from build123d import *

# Parameters (mm, degrees)
BOSS_EXTRUDE1_DEPTH = 4.7625
CUT_EXTRUDE1_DEPTH  = 3.175
FILLET1_R           = 3.302
SKETCH3_R           = 31.75
CUT_EXTRUDE2_DEPTH  = 12.7
CHAMFER1_SIZE       = 2.23064129
CHAMFER1_SIZE_2     = 2.54
SKETCH4_R           = 1.55
CUT_EXTRUDE3_DEPTH  = 50.289254661


with BuildPart() as part:
    # Sketch1 → Boss-Extrude1 (new, symmetric)
    with BuildSketch(Plane.XY):
        Polygon((-44.45, 19.05), (-44.45, -6.35), (-25.4, -6.35), (-25.4, 6.35), (-28.575, 6.35), (-28.575, 19.05), align=None)
    extrude(amount=BOSS_EXTRUDE1_DEPTH, both=True)

    # Sketch2 → Cut-Extrude1 (cut, symmetric)
    with BuildSketch(Plane.XY):
        Polygon((-44.45, 19.05), (-38.1, 19.05), (-38.1, 0), (-25.4, 0), (-25.4, -6.35), (-44.45, -6.35), align=None)
    extrude(amount=CUT_EXTRUDE1_DEPTH, both=True, mode=Mode.SUBTRACT)

    # Fillet1
    fillet1_edges = [part.edges().sort_by_distance(p)[0] for p in [
        (-38.1, 0, 0),
    ]]
    fillet(fillet1_edges, radius=FILLET1_R)

    # Sketch3 → Cut-Extrude2 (cut)
    with BuildSketch(Plane(origin=(0, 19.05, 0), x_dir=(1, 0, 0), z_dir=(0, 1, 0))):
        Circle(SKETCH3_R)
    extrude(amount=-CUT_EXTRUDE2_DEPTH, mode=Mode.SUBTRACT)

    # Chamfer1
    # the kernel refuses this chamfer: 2.54, 2.23064129 mm, written as the material it takes off along each edge
    with BuildSketch(Plane(origin=(-31.390780394, 6.35, -4.7625), x_dir=(-1, 0, 0), z_dir=(0, 1, 0))) as chamfer1_piece_1:
        with BuildLine():
            Line((CHAMFER1_SIZE, 0), (0.288027051, 2.637492029))
            ThreePointArc((0.288027051, 2.637492029), (0.17562072, 1.352980867), (0, 0))
            Line((0, 0), (CHAMFER1_SIZE, 0))
        make_face()
    extrude(amount=19.52205078, mode=Mode.SUBTRACT)
    with BuildSketch(Plane(origin=(-31.390780394, 6.35, 4.7625), x_dir=(-0.11419845391674416, 0, -0.993457957400828), z_dir=(0, 1, 0))) as chamfer1_piece_2:
        with BuildLine():
            Line((2.293129868, 0), (CHAMFER1_SIZE_2 * 0.114198453917, CHAMFER1_SIZE_2 * 0.993457957401))
            Line((CHAMFER1_SIZE_2 * 0.114198453917, CHAMFER1_SIZE_2 * 0.993457957401), (0, 0))
            ThreePointArc((0, 0), (1.178209116, 0.020693522), (2.293129868, 0))
        make_face()
    extrude(amount=19.232074789, mode=Mode.SUBTRACT)
    with BuildSketch(Plane(origin=(0, 19.05, 0), x_dir=(-0.9371917542835735, 0, -0.34881458642504903), z_dir=(0.34881458642504903, 0, -0.9371917542835735))) as chamfer1_piece_3:
        Polygon((31.75, -CHAMFER1_SIZE_2), (31.75 + CHAMFER1_SIZE_2, 0), (31.75, 0), align=None)
    revolve(axis=Axis((0, 19.05, 0), (0, 1, 0)), revolution_arc=40.829654119, mode=Mode.SUBTRACT)

    # Sketch4 → Cut-Extrude3 (cut, through all)
    with BuildSketch(Plane.XY.offset(4.7625)):
        with Locations((-41.275, 5.08)):
            Circle(SKETCH4_R)
    extrude(amount=-CUT_EXTRUDE3_DEPTH, mode=Mode.SUBTRACT)


solid = part.part
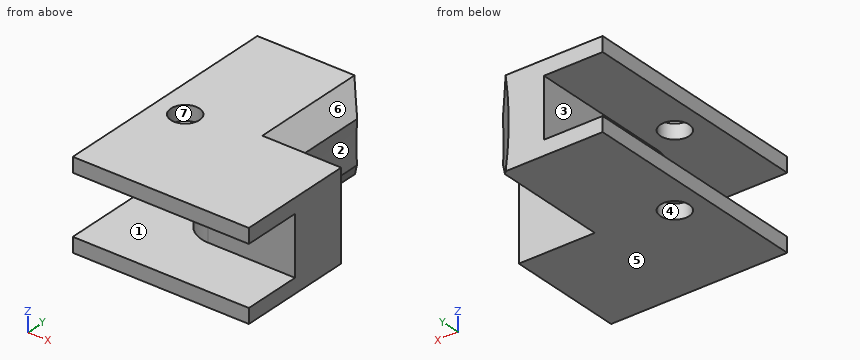
For this review, take the finished solid that the model builds, in its own axes (mm). Face numbers are marked on the shaded views. A direction names the side the tool comes from. Round coordinates to 2 decimals unless told otherwise and drop trailing zeros. Put each result on its own line as item: value. Start each with the question number.
1. For the marked faces 1, 2 and 3, list the 3-axis set-ups (+Z, -Z, +X, -X, +Y, -Y) from which the entire face can be reached by the end or side of a thin tool; tool diameter is ignored.
2. For probe 1 along Z at (x, y) = (-35, -5.25) (1 decimal); probe 2 along Y at (x, z) = (-30, -4); probe 3 along X at (y, z) = (12, 0.5), list the stretches that pass through material, from the lowest coordinate up. Write a range as [from, to].
3. Consider section B-B on y = 5.08. State how many separate pieces and enclosed holes the cut face has, plus the area to 3 significant figures.
4. Mouldability with a two-part tool opening along X and no side actions: class the marked faces 4, 5, 6 and 7 as +X half, -X half, draft (parallel to the pull), parting line (faces both ways), or undercut.
5. Insertion check: P1, Ø4.5, axis at x = -28, z = 1, coming from the +Y side; P2, Ø1.9, axis at x = -41.275, y = 5.08, coming from the -Z side; P3, Ø5, axis at x = -30, z = 0, coming from the -Y side; P4, Ø2, axis at x = -31.5, y = 16, coming from the -Z side. Each pin has a flat end and moves straight along its axis. Give the tip position at first contact, or say it passes through.
Result sheet:
1. face 1: -X, -Y
1. face 2: +X, +Y
1. face 3: -X, +Y, -Y
2. probe 1: [-4.8, -3.2], [3.2, 4.8]
2. probe 2: [-6.35, 6.35]
2. probe 3: [-38.1, -31.75]
3. separate pieces: 3
3. enclosed holes: 0
3. area: 131 mm^2
4. face 4: undercut
4. face 5: draft
4. face 6: +X half
4. face 7: undercut
5. P1: y = 6.35
5. P2: through
5. P3: y = 0
5. P4: z = -3.24
